```python
from build123d import *

# Parameters (mm, degrees)
F1_DEPTH = 57.15
F0_R     = 6.35
F2_DEPTH = 25.4
F4_DEPTH = 63.501


with BuildPart() as f1:
    # F0 (on Front) → F1 (new body)
    with BuildSketch(Plane.XZ):
        Polygon((0, 6.35), (0, 0), (38.1, 0), (38.1, 12.7), (50.8, 12.7), (50.8, 19.05), (38.1, 19.05), (38.1, 31.75), (-6.35, 31.75), (-6.35, 6.35), align=None)
    extrude(amount=F1_DEPTH)

    # F0 (on Front) → F2 (join)
    with BuildSketch(Plane.XZ):
        Polygon((-6.35, 63.5), (-6.35, 31.75), (38.1, 31.75), (38.1, 19.05), (50.8, 19.05), (50.8, 12.7), (101.6, 12.7), (101.6, 31.75), (44.45, 63.5), align=None)
        with Locations((12.7, 50.8)):
            Circle(F0_R, mode=Mode.SUBTRACT)
    extrude(amount=F2_DEPTH)

    # F3 (on face) → F4 (cut, through all)
    with BuildSketch(Plane.XY.offset(63.5)):
        Polygon((101.6, 0), (85.725, 0), (101.6, -15.875), align=None)
    extrude(amount=-F4_DEPTH, mode=Mode.SUBTRACT)


solid = f1.part
```
Geometry: final body of the model. Coordinates: model frame, mm. A direction names the side the tool comes from. Round coordinates to 2 decimals unless told otherwise and drop trailing zeros. Write each loop counter-clockwise with the first axis right and the second up, starting at its lowest first coordinate (ties: lowest second). Pieces come first, ordered by that corner, then holes. Notation, with made-up numbers: M 16,39.25 L 20,39.25 A10 cw 20,48.25 Z; hole C 82,54.25 d10. An arc over 180 degrees is marked long. Answer in a Markdown table with one row per item. Add a question column.
(1) Contact query for flat-ended pins moving along their axis: pin 1 (10 mm diameter, centred on x = 45, y = -45.5, fed in from +Z); pin 2 (14 mm diameter, centred on y = -48.5, z = 23.5, fed in from +X); pin 3 (6 mm diameter, centred on y = -15.5, z = 14.5, fed in from +X); pin 4 (5 mm diameter, centred on x = -4.5, y = -16.5, fed in from -Z). Output: stop coordinate, or through.
(2) Reachability of faces 4 (the face through (38.1, -28, 6)), 5 (the face through (-3, -28, 6.35)), 6 (the face through (45, -41, 19.05)) from +Z, -Z, +X, -X, +Y, -Y: full face, straight path, thin tool, end or side. Return the list, or none.
(3) Cut plane A-A, the plane x = 12.7. Return the cut outline in (y, z), then the cut area to 3 significant figures.
(4) Cut plane B-B, the plane y = -21. Return the cut outline in (x, z), then the cut area to 3 significant figures.
(5) Cut plane D-D, the plane z = 26.5. Return the cut outline in (x, y) (3 decimals), then the cut area to 3 significant figures.
(6) Draft query along Z for faces 1 (the face through (19, -13, 63.5)), 2 (the face through (11.9, -12.5, 57.1)), 3 (the face through (50.8, -41, 16)). Return one class per face: pulls with the +Z half, pulls with the -Z half, needs draft (parallel to the pull), parting line crosses it, or undercut.
(7) Cut plane C-C, the plane z = 50.8. Return the cut outline in (x, y).
(8) Ray query, L1, parallel to Z at x = 12.7, y = -17; L2, parallel to X at y = -10, z = 8; L3, parallel to Y at x = 56.5, z = 48. Return the intervals inside material, ascending.
Established:
| question | item | result |
|---|---|---|
| 1 | pin 1 | z = 19.05 |
| 1 | pin 2 | x = 50.8 |
| 1 | pin 3 | x = 101.6 |
| 1 | pin 4 | z = 6.35 |
| 2 | face 4 | -Z, +X, +Y, -Y |
| 2 | face 5 | -Z, -X, +Y, -Y |
| 2 | face 6 | +Z, +X, -Y |
| 3 | outline | M -57.15,0 L 0,0 L 0,44.45 L -25.4,44.45 L -25.4,31.75 L -57.15,31.75 Z; M -25.4,57.15 L 0,57.15 L 0,63.5 L -25.4,63.5 Z |
| 3 | area | 2,300 mm² |
| 4 | outline | M -6.35,6.35 L 0,6.35 L 0,0 L 38.1,0 L 38.1,12.7 L 101.6,12.7 L 101.6,31.75 L 44.45,63.5 L -6.35,63.5 Z; hole C 12.7,50.8 d12.7 |
| 4 | area | 4,970 mm² |
| 5 | outline | M -6.35,-57.15 L 38.1,-57.15 L 38.1,-25.4 L 101.6,-25.4 L 101.6,-15.875 L 85.725,0 L -6.35,0 Z |
| 5 | area | 4,030 mm² |
| 6 | face 1 | pulls with the +Z half |
| 6 | face 2 | undercut |
| 6 | face 3 | needs draft |
| 7 | outline | M -6.35,-25.4 L 6.35,-25.4 L 6.35,0 L -6.35,0 Z; M 19.05,-25.4 L 67.31,-25.4 L 67.31,0 L 19.05,0 Z |
| 8 | L1 | 0 to 44.45, 57.15 to 63.5 |
| 8 | L2 | -6.35 to 38.1 |
| 8 | L3 | -25.4 to 0 |
